Solid Edge part; units mm, degrees
sketch "Sketch1" plane through (0, 0, 0) normal (0, 0, 1) x (1, 0, 0)
  circle A0 centre (20, 0) radius 1
  circle A1 centre (0, 0) radius 0.5
  circle A2 centre (-20, 0) radius 1
  circle A3 centre (0, 0) radius 36.21
extrude "Protrusion1" add sketch "Sketch1" against normal blind 3
chamfer "Chamfer_1" distance 1.5 angle 45 2 edges at (19, 0, 0) (-21, 0, 0)
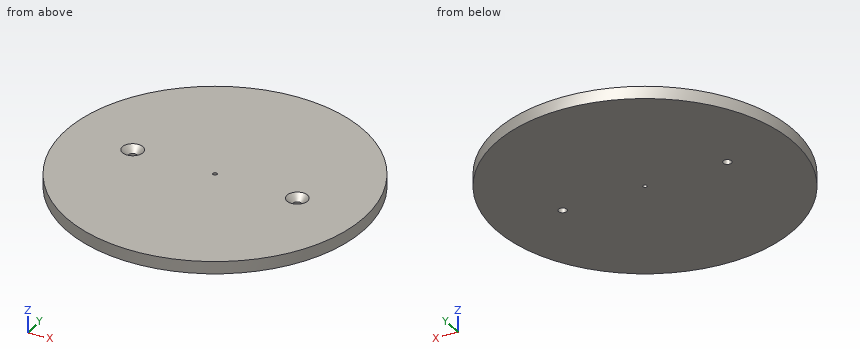
The listing builds one solid part. Answer for the finished solid, in the listing's coordinates (mm). Round coordinates to 2 decimals unless told otherwise and drop trailing zeros. Order: outer loops, then holes, each group sorted by start corner. A loop starts at its lowest first (then second) coordinate and runs counter-clockwise, first axis right, second up. Notation, with made-up numbers: (-17, 71) -> (40, 71) arc R15 ccw to (40, 89) -> close; hole circle Ø4 at (4, 43). An arc over 180 degrees is marked (long way). One line per item, written item: value.
Item 1: Find section C-C, the plane y = -13. Give the vertices of the cut face in (x, z), then the cut area to 3 significant figures.
Taken from the geometry:
outline: (-33.8, -3) -> (33.8, -3) -> (33.8, 0) -> (-33.8, 0) -> close
area: 203 mm2
Item 2: Given P1, Ø1, axis at x = 23.5, z = -2, coming from the +Y side; P2, Ø1.5, axis at x = 1, z = -2.5, coming from the -Y side; P3, Ø1.5, axis at x = -18.5, z = -1.5, coming from the +Y side, each flat-ended and moving along its own axis, determine where each tip first touches the part or whether it passes through.
Taken from the geometry:
P1: stops at y = 27.97
P2: stops at y = -36.21
P3: stops at y = 31.56
Item 3: Straight lines are drawn through the part: L1, parallel to Y at x = 20, z = -2.15; L2, parallel to X at y = -21, z = -0.55; L3, parallel to X at y = 26.5, z = -0.05. For each, find the intervals that lie inside material, in ascending order.
Taken from the geometry:
L1: y = -30.19 to -1, 1 to 30.19
L2: x = -29.5 to 29.5
L3: x = -24.68 to 24.68
Item 4: Find section D-D, the plane x = 11. Give the vertices of the cut face in (y, z).
Taken from the geometry:
outline: (-34.5, -3) -> (34.5, -3) -> (34.5, 0) -> (-34.5, 0) -> close
Item 5: Find section A-A, the plane x = -20. Give the vertices of the cut face in (y, z).
Taken from the geometry:
outline: (-30.19, -3) -> (-1, -3) -> (-1, -1.5) -> (-2.5, 0) -> (-30.19, 0) -> close; (1, -3) -> (30.19, -3) -> (30.19, 0) -> (2.5, 0) -> (1, -1.5) -> close
Item 6: Find section B-B, the plane z = -2.3. Give the vertices of the cut face in (x, y).
Taken from the geometry:
outline: circle Ø72.42 at (0, 0); hole circle Ø2 at (-20, 0); hole circle Ø1 at (0, 0); hole circle Ø2 at (20, 0)
